Job drawing, mm, ordinate dimensions from the low corner. One solid piece. Give positions to 0.01 mm unless a question says otherwise; leave off trailing zeros. Write each loop counter-clockwise with the first axis right and the second up, starting at its lowest first coordinate (ties: lowest second). Pieces come first, ordered by that corner, then holes. Notation, with made-up numbers: (6.25, 62) - (31.25, 62) arc R25 cw to (31.25, 82) - close; hole circle Ø2 at (35, 50.25). An arc over 180 degrees is marked (long way). Use a Markdown table: item, result. Add a question column.
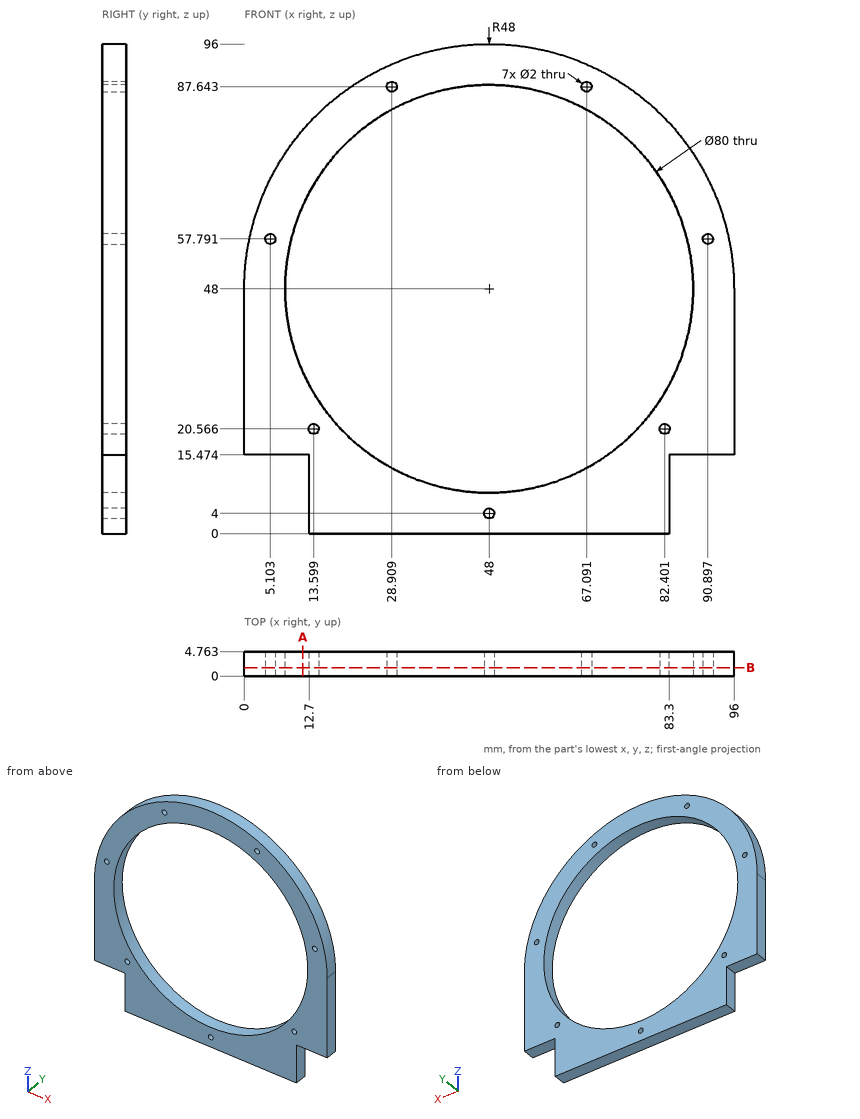
(1) Probe probe 1 along Z at (x, y) = (48, 3.1); probe 2 along X at (y, z) = (1.55, 49); probe 3 along X at (y, z) = (3.5, 53.5) (1 decimal). List the from-to ranges inside material, lowest first. Write a range as [from, to].
(2) Band-saw the part on A-A (x = 11.5). Write the cut outline in (y, z) (1 decimal).
(3) Band-saw the part on B-B (y = 1.65). Give the number of separate pieces and of enclosed holes in the cut face.
(4) Flat gauge pins, fed straight in: pin 1 (1.5 mm diameter, centred on x = 60.5, y = 0.5, fed in from +Z); pin 2 (1.6 mm diameter, centred on x = 82.4, z = 20.57, fed in from -Y); pin 3 (1.4 mm diameter, centred on y = 3.5, z = 10.5, fed in from -X); pin 4 (1 mm diameter, centred on x = 61.5, y = 3, fed in from +Z). Where does each tip first touch, or does it go through?
Model answer:
| question | item | result |
|---|---|---|
| 1 | probe 1 | z = [0, 3], [5, 8], [88, 96] |
| 1 | probe 2 | x = [0.01, 8.01], [87.99, 95.99] |
| 1 | probe 3 | x = [0.3, 8.4], [87.6, 95.7] |
| 2 | outline | (0, 15.5) - (4.8, 15.5) - (4.8, 31.6) - (0, 31.6) - close; (0, 64.4) - (4.8, 64.4) - (4.8, 79.2) - (0, 79.2) - close |
| 3 | separate pieces | 1 |
| 3 | enclosed holes | 8 |
| 4 | pin 1 | stops at z = 94.54 |
| 4 | pin 2 | passes through |
| 4 | pin 3 | stops at x = 12.7 |
| 4 | pin 4 | stops at z = 94.21 |
